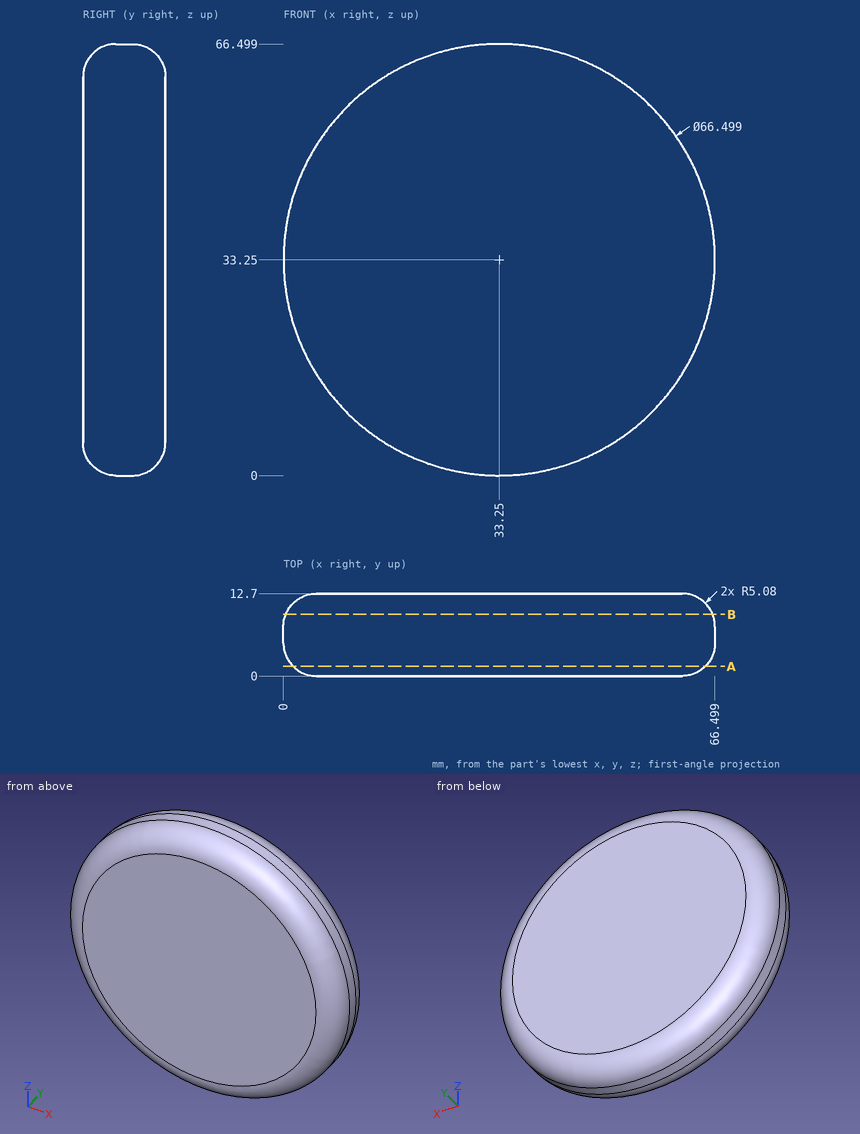
Check sheet for the drawn part. Datum: minimum x, y, z corner. Units: mm. Coordinates: 2 decimals unless noted, no trailing zeros. Order: outer loops, then holes, each group sorted by start corner. A loop starts at its lowest first (then second) coordinate and runs counter-clockwise, first axis right, second up. Notation, with made-up numbers: (70.5, -1.5) - (99.5, -1.5) arc R9 cw to (99.5, 11.5) - close; hole circle Ø7 at (61, 63). An arc over 180 degrees is marked (long way). Return JSON: item names as keys, results as strings.
(1) Go/stop test with flat-tipped pins: pin 1 (3 mm diameter, centred on y = 9.5, z = 11, fed in from -X); pin 2 (1.5 mm diameter, centred on x = 58.5, y = 1.5, fed in from -Z) (1 decimal); pin 3 (3 mm diameter, centred on y = 5, z = 46, fed in from -X). Record where each tip stops, or that it passes through.
Filled sheet:
{"pin 1": "stops at x = 7.58", "pin 2": "stops at z = 12.6", "pin 3": "stops at x = 1.96"}
(2) Thickness scan on line 1 along Z through (x, y) = (36, 6.25) (1 decimal); line 2 along Y through (x, z) = (50, 6.5); line 3 along Z through (x, y) = (4.5, 8.5) (1 decimal). Record the ranges inside material, lowest first.
Filled sheet:
{"line 1": "z = 0.1 to 66.4", "line 2": "y = 1.3 to 11.4", "line 3": "z = 16.7 to 49.8"}
(3) Section check B-B, the plane y = 9.5. Record the cut outline in (x, z).
Filled sheet:
{"outline": "circle Ø65.78 at (33.25, 33.25)"}
(4) Section check A-A, the plane y = 1.5. Record the cut outline in (x, z).
Filled sheet:
{"outline": "circle Ø63.55 at (33.25, 33.25)"}
